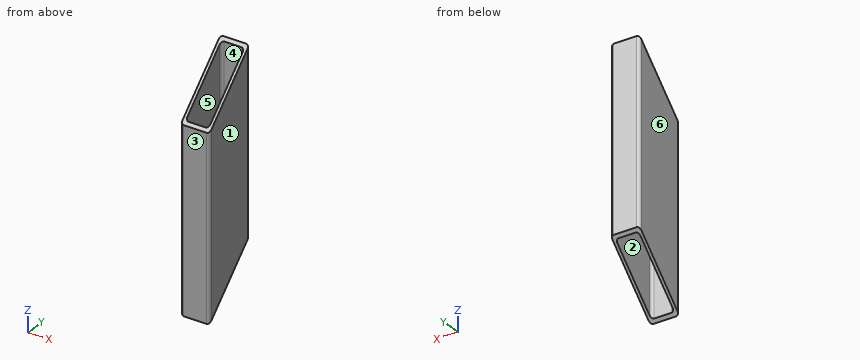
```python
from build123d import *

# Parameters (mm, degrees)
EXTRUDE_1_DEPTH     = 205.56
CUT_EXTRUDE_1_DEPTH = 50


with BuildPart() as part:
    # Эскиз1 → Бобышка-Вытянуть1 (new body)
    with BuildSketch(Plane.XY):
        with BuildLine():
            Line((-10, 50), (10, 50))
            ThreePointArc((10, 50), (11.767766953, 49.267766953), (12.5, 47.5))
            Line((12.5, 47.5), (12.5, 2.5))
            ThreePointArc((12.5, 2.5), (11.767766953, 0.732233047), (10, 0))
            Line((10, 0), (-10, 0))
            ThreePointArc((-10, 0), (-11.767766953, 0.732233047), (-12.5, 2.5))
            Line((-12.5, 2.5), (-12.5, 47.5))
            ThreePointArc((-12.5, 47.5), (-11.767766953, 49.267766953), (-10, 50))
        make_face()
        with BuildLine():
            Line((-7.5, 47.5), (7.5, 47.5))
            ThreePointArc((7.5, 47.5), (9.267766953, 46.767766953), (10, 45))
            Line((10, 45), (10, 5))
            ThreePointArc((10, 5), (9.267766953, 3.232233047), (7.5, 2.5))
            Line((7.5, 2.5), (-7.5, 2.5))
            ThreePointArc((-7.5, 2.5), (-9.267766953, 3.232233047), (-10, 5))
            Line((-10, 5), (-10, 45))
            ThreePointArc((-10, 45), (-9.267766953, 46.767766953), (-7.5, 47.5))
        make_face(mode=Mode.SUBTRACT)
    extrude(amount=-EXTRUDE_1_DEPTH)

    # Эскиз2 → Вырез-Вытянуть1 (cut)
    with BuildSketch(Plane.ZY.offset(12.5)):
        Polygon((-205.56, 50), (-155.559999999, 50), (-205.56, 0), align=None)
        Polygon((0.003491861, 0), (-49.996508139, 0), (0.003491861, 49.999999999), align=None)
    extrude(amount=-CUT_EXTRUDE_1_DEPTH, mode=Mode.SUBTRACT)


solid = part.part
```
The listing builds one solid part. Answer for the finished solid, in the listing's coordinates (mm). Face numbers are marked on the shaded views. A direction names the side the tool comes from. Coordinates: 2 decimals unless noted, no trailing zeros. Loops run counter-clockwise (first coordinate to the right, second up) from the corner with the lowest first, then second, coordinate; pieces in that order, holes last. Notation, with made-up numbers: (76.5, 83.5) - (135.5, 83.5) arc R32 ccw to (135.5, 112.5) - close; hole circle Ø2 at (-18.75, 79). An arc over 180 degrees is marked (long way). Use a Markdown table: item, result. Add a question column.
1) For the marked faces 1 and 2, determine the directions among +Z, -Z, +X, -X, +Y, -Y from which every point of the face is accessible in a straight line to the end or side of a thin tool.
2) Find the intervals of material crossed by line 1 (X direction, y = 41, z = -156.5); line 2 (Y direction, x = -6, z = -121); line 3 (Y direction, x = 3.5, z = -35.5), in increasing order.
3) The part is cut by section B-B, the plane y = 14.5. Give the vertices of the cut face in (x, z).
4) The part is cut by section D-D, the plane z = -179.5. Give the vertices of the cut face in (x, y), and give its area (3 significant figures).
5) The mould has two halves that part along Y. Classify the marked faces 3, 4, 5 and 6: released by +Y, released by -Y, zero draft, split by the parting line, or undercut.
6) The part is cut by section C-C, the plane z = -73.5. Give the vertices of the cut face in (x, y).
Here are the results:
| question | item | result |
|---|---|---|
| 1 | face 1 | +Z, -Z, +X, +Y, -Y |
| 1 | face 2 | +Z, -Z |
| 2 | line 1 | x = -12.5 to -10, 10 to 12.5 |
| 2 | line 2 | y = 0 to 2.5, 47.5 to 50 |
| 2 | line 3 | y = 47.5 to 50 |
| 3 | outline | (-12.5, -191.06) - (-10, -191.06) - (-10, -35.5) - (-12.5, -35.5) - close; (10, -191.06) - (12.5, -191.06) - (12.5, -35.5) - (10, -35.5) - close |
| 4 | outline | (-12.5, 2.5) arc R2.5 ccw to (-10, 0) - (10, 0) arc R2.5 ccw to (12.5, 2.5) - (12.5, 26.06) - (10, 26.06) - (10, 5) arc R2.5 cw to (7.5, 2.5) - (-7.5, 2.5) arc R2.5 cw to (-10, 5) - (-10, 26.06) - (-12.5, 26.06) - close |
| 4 | area | 180 mm^2 |
| 5 | face 3 | released by -Y |
| 5 | face 4 | undercut |
| 5 | face 5 | undercut |
| 5 | face 6 | zero draft |
| 6 | outline | (-12.5, 2.5) arc R2.5 ccw to (-10, 0) - (10, 0) arc R2.5 ccw to (12.5, 2.5) - (12.5, 47.5) arc R2.5 ccw to (10, 50) - (-10, 50) arc R2.5 ccw to (-12.5, 47.5) - close; hole (-10, 5) arc R2.5 ccw to (-7.5, 2.5) - (7.5, 2.5) arc R2.5 ccw to (10, 5) - (10, 45) arc R2.5 ccw to (7.5, 47.5) - (-7.5, 47.5) arc R2.5 ccw to (-10, 45) - close |
